from build123d import *

# Parameters (mm, degrees)
BOSS_EXTRUDE1_DEPTH     = 111.76
SKETCH5_W               = 304.8
SKETCH5_H               = 25.4
CUT_EXTRUDE3_DEPTH      = 101.6
CUT_EXTRUDE4_DEPTH      = 227.288199427
CUT_EXTRUDE4_DEPTH_BACK = 227.288199427
SKETCH3_W               = 96.52
SKETCH3_H               = 101.6
SKETCH3_W_2             = 48.26
CUT_EXTRUDE5_REACH      = 288.663
SKETCH6_W               = 38.1
SKETCH6_H               = 50.8
SKETCH7_W               = 81.28
SKETCH7_H               = 50.8
BOSS_EXTRUDE2_DEPTH     = 5.08


with BuildPart() as part:
    # Sketch1 → Boss-Extrude1 (new body)
    with BuildSketch(Plane.XY):
        Polygon((-152.4, 62.23), (-152.4, -33.02), (0, -62.23), (152.4, -32.976439839), (152.4, 62.23), align=None)
    extrude(amount=-BOSS_EXTRUDE1_DEPTH)

    # Sketch5 → Cut-Extrude3 (cut)
    with BuildSketch(Plane.XY.offset(-5.08)):
        with Locations((0, -1.27)):
            Rectangle(SKETCH5_W, SKETCH5_H)
    extrude(amount=-CUT_EXTRUDE3_DEPTH, mode=Mode.SUBTRACT)

    # Sketch3 → Cut-Extrude4 (cut, two sides: drawn at the far end of the back side and taken through both)
    with BuildSketch(Plane(origin=(0, 62.23, 0), x_dir=(1, 0, 0), z_dir=(0, 1, 0)).offset(-CUT_EXTRUDE4_DEPTH_BACK)):
        with Locations((-50.8, 55.88)):
            Rectangle(SKETCH3_W, SKETCH3_H)
        with Locations((50.8, 55.88)):
            Rectangle(SKETCH3_W, SKETCH3_H)
        with Locations((-128.27, 55.88)):
            Rectangle(SKETCH3_W_2, SKETCH3_H)
        with Locations((128.27, 55.88)):
            Rectangle(SKETCH3_W_2, SKETCH3_H)
    extrude(amount=CUT_EXTRUDE4_DEPTH + CUT_EXTRUDE4_DEPTH_BACK, mode=Mode.SUBTRACT)

    # Cut-Extrude5: up to this face of the body (flat: up to its plane)
    cut_extrude5_end = Plane(part.part.faces().sort_by_distance((104.14, 36.83, -55.88))[0])
    # Sketch6 → Cut-Extrude5 (cut, up to the picked face)
    with BuildSketch(Plane.ZY.offset(104.14), mode=Mode.PRIVATE) as cut_extrude5_sk1:
        with Locations((-55.932057734, 36.83)):
            Rectangle(SKETCH6_W, SKETCH6_H)
    cut_extrude5_tool1 = split(extrude(cut_extrude5_sk1.sketch, amount=-CUT_EXTRUDE5_REACH, mode=Mode.PRIVATE), bisect_by=cut_extrude5_end, keep=Keep.BOTH, mode=Mode.PRIVATE)
    add(cut_extrude5_tool1.solids().sort_by(Axis((-104.14, 36.83, -55.932058), (1, 0, 0)))[0], mode=Mode.SUBTRACT)

    # Sketch7 → Boss-Extrude2 (add)
    with BuildSketch(Plane(origin=(0, 0, -36.882057734), x_dir=(-1, 0, 0), z_dir=(0, 0, -1))):
        with Locations((0, 36.83)):
            Rectangle(SKETCH7_W, SKETCH7_H)
        with Locations((101.6, 36.83)):
            Rectangle(SKETCH7_W, SKETCH7_H)
        with Locations((-101.6, 36.83)):
            Rectangle(SKETCH7_W, SKETCH7_H)
    boss_extrude2 = extrude(amount=-BOSS_EXTRUDE2_DEPTH)

    # Mirror1: Boss-Extrude2 across plane
    add(boss_extrude2.mirror(Plane(origin=(0, 0, -55.932057734), x_dir=(1, 0, 0), z_dir=(0, 0, -1))))


solid = part.part
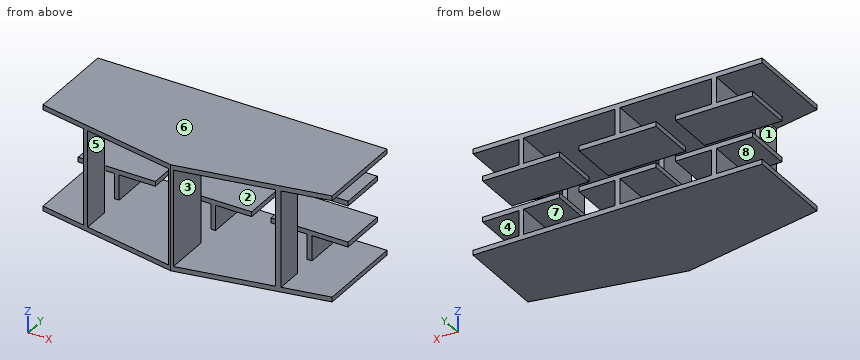
The model under review builds one solid part; all positions refer to its coordinate system, in mm. Face numbers are marked on the shaded views. A direction names the side the tool comes from. Give positions to 0.01 mm unless a question says otherwise; leave off trailing zeros. Write each loop counter-clockwise with the first axis right and the second up, starting at its lowest first coordinate (ties: lowest second). Pieces come first, ordered by that corner, then holes.
1. Add section C-C, the plane y = -8.5. Write out the cut boundary in (x, z).
2. Wall thickness on L1, parallel to Z at x = 10, y = 34; L2, parallel to X at y = -21.5, z = -50; L3, parallel to X at y = 29.5, z = -78.5: over which ranges is each line inside the solid? List them lowest first.
3. For P1, Ø23.5, axis at y = -34.5, z = -48.5, coming from the +X side; P2, Ø1, axis at y = -46, z = -71, coming from the -X side; P3, Ø5.5, axis at y = 45, z = -34.5, coming from the +X side, all flat-tipped, find the tip position at first contact; note any pin that passes through.
4. Add section A-A, the plane z = -64. Write out the cut boundary in (x, y), plus the area to 3 significant figures.
5. Add section B-B, the plane z = -13. Write out the cut boundary in (x, y).
6. Draft analysis for pull direction X (two halves, no side actions). For the marked faces 1, 2 and 3, state which applies: +X half, -X half, draft (parallel to the pull), parting line (faces both ways), or undercut.
7. Tool access review of the marked faces 4, 5, 6, 7 and 8: name each direction out of +Z, -Z, +X, -X, +Y, -Y from which nothing blocks a thin tool from reaching the whole face with its end or side.
8. Add section D-D, the plane x = -89. Write out the cut boundary in (y, z).
Worked answers:
1. outline: (-152.4, -111.76) - (152.4, -111.76) - (152.4, -106.68) - (-152.4, -106.68) - close; (-152.4, -5.08) - (152.4, -5.08) - (152.4, 0) - (-152.4, 0) - close
2. L1: z = -111.76 to -106.68, -80.06 to -74.98, -36.88 to -31.8, -5.08 to 0
2. L2: x = -104.14 to -99.06, -2.54 to 2.54, 99.06 to 104.14
2. L3: x = -142.24 to -60.96, -40.64 to 40.64, 60.96 to 142.24
3. P1: stops at x = 104.14
3. P2: stops at x = -2.54
3. P3: stops at x = 142.24
4. outline: (-104.14, -42.27) - (-99.06, -43.24) - (-99.06, -13.97) - (-104.14, -13.97) - close; (-2.54, -61.74) - (0, -62.23) - (2.54, -61.74) - (2.54, -13.97) - (-2.54, -13.97) - close; (99.06, -43.22) - (104.14, -42.24) - (104.14, -13.97) - (99.06, -13.97) - close
4. area: 536 mm2
5. outline: (-104.14, -42.27) - (-99.06, -43.24) - (-99.06, -13.97) - (-104.14, -13.97) - close; (-104.14, 11.43) - (-99.06, 11.43) - (-99.06, 62.23) - (-104.14, 62.23) - close; (-2.54, -61.74) - (0, -62.23) - (2.54, -61.74) - (2.54, -13.97) - (-2.54, -13.97) - close; (-2.54, 11.43) - (2.54, 11.43) - (2.54, 62.23) - (-2.54, 62.23) - close; (99.06, -43.22) - (104.14, -42.24) - (104.14, -13.97) - (99.06, -13.97) - close; (99.06, 11.43) - (104.14, 11.43) - (104.14, 62.23) - (99.06, 62.23) - close
6. face 1: -X half
6. face 2: draft
6. face 3: undercut
7. face 4: +X, +Y, -Y
7. face 5: -Y
7. face 6: +Z, +X, -X, +Y, -Y
7. face 7: +Y, -Y
7. face 8: -X, +Y, -Y
8. outline: (-45.17, -111.76) - (62.23, -111.76) - (62.23, -106.68) - (-45.17, -106.68) - close; (-45.17, -5.08) - (62.23, -5.08) - (62.23, 0) - (-45.17, 0) - close; (11.43, -80.06) - (62.23, -80.06) - (62.23, -74.98) - (11.43, -74.98) - close; (11.43, -36.88) - (62.23, -36.88) - (62.23, -31.8) - (11.43, -31.8) - close
